The listing builds one solid part. Answer for the finished solid, in the listing's coordinates (mm). A direction names the side the tool comes from. Round coordinates to 2 decimals unless told otherwise and drop trailing zeros. Write each loop counter-clockwise with the first axis right and the second up, starting at its lowest first coordinate (ties: lowest second). Pieces come first, ordered by that corner, then holes.
from build123d import *

# Parameters (mm, degrees)
BASE_TRIANGLE_DEPTH   = 8
SKETCH2_W             = 50
SKETCH2_H             = 8
RECTANGLE_BLOCK_DEPTH = 38
CUT_EXTRUDE2_REACH    = 17.365
SKETCH3_W             = 38
SKETCH3_H             = 18
CYINDER_BLOCK_DEPTH   = 50
CUT_EXTRUDE3_REACH    = 68.918
SKETCH5_R             = 6
BOSS_EXTRUDE5_DEPTH   = 50
CUT_EXTRUDE4_DEPTH    = 50
SKETCH11_R            = 6
CUT_EXTRUDE5_DEPTH    = 50
CUT_EXTRUDE6_REACH    = 17.365
SKETCH12_W            = 38
SKETCH12_H            = 17.507702416
BOSS_EXTRUDE6_DEPTH   = 38
CUT_EXTRUDE7_REACH    = 48
SKETCH14_R            = 9
CUT_EXTRUDE9_REACH    = 10
BOSS_EXTRUDE7_DEPTH   = 22


with BuildPart() as part:
    # Sketch1 → Base triangle (new body)
    with BuildSketch(Plane(origin=(0, 0, 0), x_dir=(1, 0, 0), z_dir=(0, 1, 0))):
        with BuildLine():
            Line((0, -54.608695652), (0, 45.391304348))
            Line((0, 45.391304348), (66.917901683, 45.391304348))
            ThreePointArc((66.917901683, 45.391304348), (80, 37.730153279), (79.71890745, 22.572464832))
            Line((79.71890745, 22.572464832), (27.801005766, -62.427535168))
            ThreePointArc((27.801005766, -62.427535168), (10.938909413, -69.048485929), (0, -54.608695652))
        make_face()
    extrude(amount=BASE_TRIANGLE_DEPTH)

    # Sketch2 → Rectangle Block (add)
    with BuildSketch(Plane(origin=(0, 8, 0), x_dir=(1, 0, 0), z_dir=(0, 1, 0))):
        with Locations((40, 34.025974009)):
            Rectangle(SKETCH2_W, SKETCH2_H)
    extrude(amount=RECTANGLE_BLOCK_DEPTH)

    # Sketch3 → Cut-Extrude2 (cut, up to next)
    with BuildSketch(Plane.XY.offset(-30.025974009), mode=Mode.PRIVATE) as cut_extrude2_sk1:
        with Locations((40, 25)):
            Rectangle(SKETCH3_W, SKETCH3_H)
    cut_extrude2_tool1 = extrude(cut_extrude2_sk1.sketch, amount=-CUT_EXTRUDE2_REACH, mode=Mode.PRIVATE) & part.part
    add(cut_extrude2_tool1.solids().sort_by_distance((40, 25, -30.025974))[0], mode=Mode.SUBTRACT)

    # Sketch4 → Cyinder Block (add)
    with BuildSketch(Plane.ZY.offset(-15)):
        with BuildLine():
            ThreePointArc((-24.025974009, 55.16515139), (-39.503199584, 63.531751655), (-38.025974009, 46))
            Line((-38.025974009, 46), (-30.025974009, 46))
            ThreePointArc((-30.025974009, 46), (-25.659373744, 49.687925815), (-24.025974009, 55.16515139))
        make_face()
        with BuildLine():
            Line((-30.025974009, 46), (-38.025974009, 46))
            ThreePointArc((-38.025974009, 46), (-34.025974009, 45.16515139), (-30.025974009, 46))
        make_face()
    extrude(amount=-CYINDER_BLOCK_DEPTH)

    # Sketch5 → Cut-Extrude3 (cut, up to next)
    with BuildSketch(Plane.ZY.offset(-15), mode=Mode.PRIVATE) as cut_extrude3_sk1:
        with Locations((-34.025974009, 55.16515139)):
            Circle(SKETCH5_R)
    cut_extrude3_tool1 = extrude(cut_extrude3_sk1.sketch, amount=-CUT_EXTRUDE3_REACH, mode=Mode.PRIVATE) & part.part
    add(cut_extrude3_tool1.solids().sort_by_distance((15, 55.165151, -34.025974))[0], mode=Mode.SUBTRACT)

    # Sketch9 → Boss-Extrude5 (add)
    with BuildSketch(Plane(origin=(65, 0, 0), x_dir=(0, 0, -1), z_dir=(1, 0, 0))):
        with BuildLine():
            Line((30.025974009, 8), (38.025974009, 8))
            Line((38.025974009, 8), (38.025974009, 38.83484861))
            ThreePointArc((38.025974009, 38.83484861), (34.025974009, 58), (30.025974009, 38.83484861))
            Line((30.025974009, 38.83484861), (30.025974009, 8))
        make_face()
    extrude(amount=-BOSS_EXTRUDE5_DEPTH)

    # Sketch10 → Cut-Extrude4 (cut)
    with BuildSketch(Plane(origin=(65, 0, 0), x_dir=(0, 0, -1), z_dir=(1, 0, 0))):
        with BuildLine():
            ThreePointArc((43.362201908, 51.582575695), (34.025974009, 58), (24.68974611, 51.582575695))
            ThreePointArc((24.68974611, 51.582575695), (34.025974009, 65.16515139), (43.362201908, 51.582575695))
        make_face()
    extrude(amount=-CUT_EXTRUDE4_DEPTH, mode=Mode.SUBTRACT)

    # Sketch11 → Cut-Extrude5 (cut)
    with BuildSketch(Plane(origin=(65, 0, 0), x_dir=(0, 0, -1), z_dir=(1, 0, 0))):
        with Locations((34.025974009, 48)):
            Circle(SKETCH11_R)
    extrude(amount=-CUT_EXTRUDE5_DEPTH, mode=Mode.SUBTRACT)

    # Sketch12 → Cut-Extrude6 (cut, up to next)
    with BuildSketch(Plane.XY.offset(-30.025974009), mode=Mode.PRIVATE) as cut_extrude6_sk1:
        with Locations((40, 24.753851208)):
            Rectangle(SKETCH12_W, SKETCH12_H)
    cut_extrude6_tool1 = extrude(cut_extrude6_sk1.sketch, amount=-CUT_EXTRUDE6_REACH, mode=Mode.PRIVATE) & part.part
    add(cut_extrude6_tool1.solids().sort_by_distance((40, 24.753851, -30.025974))[0], mode=Mode.SUBTRACT)

    # Sketch13 → Boss-Extrude6 (add)
    with BuildSketch(Plane(origin=(0, 8, 0), x_dir=(1, 0, 0), z_dir=(0, 1, 0))):
        with BuildLine():
            ThreePointArc((30, -54.608695652), (15, -39.608695652), (0, -54.608695652))
            ThreePointArc((0, -54.608695652), (10.938909413, -69.048485929), (27.801005766, -62.427535168))
            ThreePointArc((27.801005766, -62.427535168), (29.439790277, -58.669786239), (30, -54.608695652))
        make_face()
    extrude(amount=BOSS_EXTRUDE6_DEPTH)

    # Sketch14 → Cut-Extrude7 (cut, up to next)
    with BuildSketch(Plane(origin=(0, 46, 0), x_dir=(1, 0, 0), z_dir=(0, 1, 0)), mode=Mode.PRIVATE) as cut_extrude7_sk1:
        with Locations((15, -54.608695652)):
            Circle(SKETCH14_R)
    cut_extrude7_tool1 = extrude(cut_extrude7_sk1.sketch, amount=-CUT_EXTRUDE7_REACH, mode=Mode.PRIVATE) & part.part
    add(cut_extrude7_tool1.solids().sort_by_distance((15, 46, 54.608696))[0], mode=Mode.SUBTRACT)

    # Sketch15 → Cut-Extrude9 (cut, up to next)
    with BuildSketch(Plane(origin=(0, 8, 0), x_dir=(1, 0, 0), z_dir=(0, 1, 0)), mode=Mode.PRIVATE) as cut_extrude9_sk1:
        Polygon((20, -37.108695652), (20, 5.391304348), (45.958950842, 5.391304348), align=None)
    cut_extrude9_tool1 = extrude(cut_extrude9_sk1.sketch, amount=-CUT_EXTRUDE9_REACH, mode=Mode.PRIVATE) & part.part
    add(cut_extrude9_tool1.solids().sort_by_distance((28.652984, 8, 8.775362))[0], mode=Mode.SUBTRACT)

    # Sketch20 → Boss-Extrude7 (add)
    with BuildSketch(Plane(origin=(0, 0, 0), x_dir=(-1, 0, 0), z_dir=(0, -1, 0))):
        with BuildLine():
            Line((-75.332662932, 15.391304348), (0, 15.391304348))
            Line((0, 15.391304348), (0, 45.391304348))
            Line((0, 45.391304348), (-66.917901683, 45.391304348))
            ThreePointArc((-66.917901683, 45.391304348), (-80, 37.730153279), (-79.71890745, 22.572464832))
            Line((-79.71890745, 22.572464832), (-75.332662932, 15.391304348))
        make_face()
    extrude(amount=BOSS_EXTRUDE7_DEPTH)


solid = part.part
1. Given pin 1 (9 mm diameter, centred on x = 35, y = 3.5, fed in from +Z); pin 2 (10 mm diameter, centred on x = 36.5, z = 31, fed in from -Y); pin 3 (6 mm diameter, centred on y = 22, z = -37, fed in from +X); pin 4 (2.5 mm diameter, centred on x = 32, z = -34.5, fed in from +Y), each flat-ended and moving along its own axis, determine where each tip first touches the part or whether it passes through.
Geometry says:
pin 1: stops at z = 58.01
pin 2: stops at y = 0
pin 3: stops at x = 65
pin 4: stops at y = 58
2. Section A-A on y = 48 is taken. Determine the outline of the cut face in (x, z), plus the area to 3 significant figures.
Geometry says:
outline: (15, -44.03) - (65, -44.03) - (65, -40.03) - (15, -40.03) - close; (15, -28.03) - (65, -28.03) - (65, -24.03) - (15, -24.03) - close
area: 400 mm2
3. For a pull along X with two mould halves and no side action, classify faces 6 (the face through (32, 8, -16)), 7 (the face through (79.89, -6.79, -37.92)), 8 (the face through (15, 39, -34)), 9 (the face through (21, 25, -34)) as released by +X, released by -X, zero draft, split by the parting line, or undercut.
Geometry says:
face 6: zero draft
face 7: released by +X
face 8: released by -X
face 9: undercut
4. Section D-D on x = 8 is taken. Determine the outline of the cut face in (y, z), plus the area to 3 significant figures.
Geometry says:
outline: (-22, -45.39) - (8, -45.39) - (8, 41.34) - (46, 41.34) - (46, 48.95) - (0, 48.95) - (0, -15.39) - (-22, -15.39) - close; (0, 60.27) - (46, 60.27) - (46, 67.88) - (0, 67.88) - close
area: 2,050 mm2
5. Straight lines are drawn through the part: line 1 along Y through (x, z) = (47, -9); line 2 along Z through (x, y) = (62, 38); line 3 along Z through (x, y) = (42, 47). For each, find the intervals that lie inside material, in ascending order.
Geometry says:
line 1: y = 0 to 8
line 2: z = -38.03 to -30.03
line 3: z = -43.98 to -39.94, -28.11 to -24.08
6. Section B-B on y = 31 is taken. Determine the outline of the cut face in (x, z), plus the area to 3 significant figures.
Geometry says:
outline: circle Ø30 at (15, 54.61); (15, -38.03) - (21, -38.03) - (21, -30.03) - (15, -30.03) - close; (59, -38.03) - (65, -38.03) - (65, -30.03) - (59, -30.03) - close; hole circle Ø18 at (15, 54.61)
area: 548 mm2
7. Section C-C on z = -32 is taken. Determine the outline of the cut face in (x, y), plus the area to 3 significant figures.
Geometry says:
outline: (0, -22) - (81.83, -22) - (81.83, 8) - (65, 8) - (65, 42.35) - (15, 42.35) - (15, 8) - (0, 8) - close; (15, 53.65) - (65, 53.65) - (65, 57.79) - (15, 57.79) - close; hole (21, 16) - (59, 16) - (59, 33.51) - (21, 33.51) - close
area: 3,710 mm2
8. A tool of negligible diameter and unlimited length cuts with its end or side. For faces 1 (the face through (40, 13, -38.026)), 2 (the face through (40, 16, -34)), 3 (the face through (33.16, 4.06, 15.56)), 4 (the face through (38, -11, -15.391)), 5 (the face through (40, 13, -30.026)), from which of +Z, -Z, +X, -X, +Y, -Y can it reach the whole face along a straight path? Write none if from no direction.
Geometry says:
face 1: -Z, +X, -X
face 2: -Z
face 3: +Y, -Y
face 4: +Z, +X, -X, -Y
face 5: +X, -X
